from build123d import *
from build123d.topology import SkipClean

# Parameters (mm, degrees)
ESQUISSE1_R                  = 9.5
BASE_EXTRUSION_DEPTH         = 17
BOSS_EXTRU_1_DEPTH           = 3
ENL_V_MAT_EXTRU_1_DEPTH      = 25.093567606
ENL_V_MAT_EXTRU_1_DEPTH_BACK = 25.093567606
ESQUISSE4_R                  = 2.25


with BuildPart() as part:
    # Esquisse1 → Base-Extrusion (new body)
    with BuildSketch(Plane(origin=(0, 0, 0), x_dir=(1, 0, 0), z_dir=(0, 1, 0))):
        with Locations(Location((0, 0, 0), (0, 0, 76.299766512))):
            Circle(ESQUISSE1_R)
    extrude(amount=BASE_EXTRUSION_DEPTH)

    # Esquisse2 → Boss.-Extru.1 (add)
    with SkipClean():  # the faces are left unmerged after this step: merging them gives an invalid solid
        with BuildSketch(Plane(origin=(0, 17, 0), x_dir=(-1, 0, 0), z_dir=(0, 1, 0))):
            with BuildLine():
                Line((-2.25, -9.229707471), (-2.25, 9.229707471))
                ThreePointArc((-2.25, 9.229707471), (-3.139988124, 8.966073532), (-4, 8.61684397))
                Line((-4, 8.61684397), (-4, -8.61684397))
                ThreePointArc((-4, -8.61684397), (-3.139988124, -8.966073532), (-2.25, -9.229707471))
            make_face()
        extrude(amount=BOSS_EXTRU_1_DEPTH)

    # Esquisse3 → Enlèvement de matière-Révolution1 (revolve, cut)
    with SkipClean():  # the faces are left unmerged after this step: merging them gives an invalid solid
        with BuildSketch(Plane.XY, mode=Mode.PRIVATE) as enl_vement_de_mati_re_r_volution1_sk:
            Polygon((8.5, 0), (8.5, 5), (7, 5), (7, 12.5), (8.5, 12.5), (8.5, 15), (0, 15), (0, 0), align=None)
        revolve(enl_vement_de_mati_re_r_volution1_sk.sketch.rotate(Axis((0, 0, 0), (0, 1, 0)), 90), axis=Axis((0, 0, 0), (0, 1, 0)), mode=Mode.SUBTRACT)

    # Esquisse4 → Enlèv. mat.-Extru.1 (cut, two sides: drawn at the far end of the back side and taken through both)
    with SkipClean():  # the faces are left unmerged after this step: merging them gives an invalid solid
        with BuildSketch(Plane.XY.offset(-ENL_V_MAT_EXTRU_1_DEPTH_BACK)):
            with Locations((0, 9)):
                Circle(ESQUISSE4_R)
        extrude(amount=ENL_V_MAT_EXTRU_1_DEPTH + ENL_V_MAT_EXTRU_1_DEPTH_BACK, mode=Mode.SUBTRACT)


solid = part.part
For this review, take the finished solid that the model builds, in its own axes (mm). A direction names the side the tool comes from. Give positions to 0.01 mm unless a question says otherwise; leave off trailing zeros. Loops run counter-clockwise (first coordinate to the right, second up) from the corner with the lowest first, then second, coordinate; pieces in that order, holes last.
Item 1: Take a section at D-D, the plane x = -7.5. State the section outline as (y, z) points, and give its area (3 significant figures).
Item 2: Take a section at C-C, the plane z = 0. State the section outline as (x, y) points.
Item 3: For line 1 along X through (y, z) = (2.3, 0); line 2 along Y through (x, z) = (6, 5), list the stretches that pass through material, from the lowest coordinate up.
Item 4: Take a section at A-A, the plane x = 0. State the section outline as (y, z) points, and give its area (3 significant figures).
Item 5: Insertion check: pin 1 (3 mm diameter, centred on y = 12, z = -4, fed in from +X); pin 2 (1 mm diameter, centred on x = -2, y = 9, fed in from -Z); pin 3 (1.5 mm diameter, centred on x = -1, z = -6, fed in from -Y); pin 4 (3.5 mm diameter, centred on x = 0, y = 9, fed in from -Z). Each pin has a flat end and moves straight along its axis. Give the tip position at first contact, or say it passes through.
Item 6: Draft analysis for pull direction Y (two halves, no side actions). For faces 1 (the cylindrical face through (-8.428, 2.535, 1.107)), 2 (the flat face through (-3, 17, -1)), 3 (the flat face through (-7, 12.5, 2)), state which applies: +Y half, -Y half, draft (parallel to the pull), parting line (faces both ways), or undercut.
Item 7: Tool access review of faces 4 (the flat face through (4, 18, 0)), 5 (the cylindrical face through (-8.428, 13.768, 1.107)), 6 (the flat face through (2.25, 18, 0)), 7 (the flat face through (-1, 0, 9)), 8 (the cylindrical face through (2.681, 8.802, -6.466)): name each direction out of +Z, -Z, +X, -X, +Y, -Y from which nothing blocks a thin tool from reaching the whole face with its end or side.
Item 8: Take a section at B-B, the plane y = 8.5. State the section outline as (x, z) points.
Calculated:
1. outline: (0, -5.83) - (17, -5.83) - (17, 5.83) - (0, 5.83) - (0, 4) - (5, 4) - (5, -4) - (0, -4) - close; hole (12.5, -4) - (15, -4) - (15, 4) - (12.5, 4) - close
1. area: 138 mm2
2. outline: (-9.5, 0) - (-8.5, 0) - (-8.5, 5) - (-7, 5) - (-7, 12.5) - (-8.5, 12.5) - (-8.5, 15) - (8.5, 15) - (8.5, 12.5) - (7, 12.5) - (7, 5) - (8.5, 5) - (8.5, 0) - (9.5, 0) - (9.5, 17) - (4, 17) - (4, 20) - (2.25, 20) - (2.25, 17) - (-9.5, 17) - close
3. line 1: x = -9.5 to -8.5, 8.5 to 9.5
3. line 2: y = 5 to 12.5, 15 to 17
4. outline: (0, -9.5) - (6.75, -9.5) - (6.75, -7) - (5, -7) - (5, -8.5) - (0, -8.5) - close; (0, 8.5) - (5, 8.5) - (5, 7) - (6.75, 7) - (6.75, 9.5) - (0, 9.5) - close; (11.25, -9.5) - (17, -9.5) - (17, 9.5) - (11.25, 9.5) - (11.25, 7) - (12.5, 7) - (12.5, 8.5) - (15, 8.5) - (15, -8.5) - (12.5, -8.5) - (12.5, -7) - (11.25, -7) - close
4. area: 68.0 mm2
5. pin 1: stops at x = 9.17
5. pin 2: stops at z = -9.24
5. pin 3: stops at y = 15
5. pin 4: passes through
6. face 1: draft
6. face 2: +Y half
6. face 3: undercut
7. face 4: +Z, -Z, +X, +Y
7. face 5: none
7. face 6: +Z, -Z, -X, +Y
7. face 7: +Z, -Z, +X, -X, -Y
7. face 8: -Y
8. outline: (-2.19, -9.24) - (-2.19, -6.65) arc R7 cw to (-2.19, 6.65) - (-2.19, 9.24) arc R9.5 ccw to start; (2.19, -9.24) arc R9.5 ccw to (2.19, 9.24) - (2.19, 6.65) arc R7 cw to (2.19, -6.65) - close
